from build123d import *

# Parameters (mm, degrees)
SKETCH1_R           = 7
BOSS_EXTRUDE1_DEPTH = 10


with BuildPart() as part:
    # Sketch1 → Boss-Extrude1 (new body)
    with BuildSketch(Plane.XY):
        with BuildLine():
            Line((-63.333523535, 182.443481279), (-143.333523535, 182.443481279))
            ThreePointArc((-143.333523535, 182.443481279), (-150.404591346, 179.514549091), (-153.333523535, 172.443481279))
            Line((-153.333523535, 172.443481279), (-153.333523535, -75.556518721))
            ThreePointArc((-153.333523535, -75.556518721), (-150.404591346, -82.627586533), (-143.333523535, -85.556518721))
            Line((-143.333523535, -85.556518721), (-63.333523535, -85.556518721))
            Line((-63.333523535, -85.556518721), (-63.333523535, 182.443481279))
        make_face()
        with Locations((-108.333523535, 48.443481279)):
            Circle(SKETCH1_R, mode=Mode.SUBTRACT)
        with Locations((-108.333523535, 123.443481279)):
            Circle(SKETCH1_R, mode=Mode.SUBTRACT)
        with Locations((-108.333523535, -26.556518721)):
            Circle(SKETCH1_R, mode=Mode.SUBTRACT)
    extrude(amount=BOSS_EXTRUDE1_DEPTH)


solid = part.part
Here's how the part is built. I have some questions about the finished solid (model axes, mm). Coordinates: 2 decimals unless noted, no trailing zeros. Order: outer loops, then holes, each group sorted by start corner. A loop starts at its lowest first (then second) coordinate and runs counter-clockwise, first axis right, second up.
Item 1: If we section it at B-B on z = 7.75: List the corners of the cut face in (x, y) for me.
Result sheet:
outline: (-153.33, -75.56) arc R10 ccw to (-143.33, -85.56) - (-63.33, -85.56) - (-63.33, 182.44) - (-143.33, 182.44) arc R10 ccw to (-153.33, 172.44) - close; hole circle Ø14 at (-108.33, -26.56); hole circle Ø14 at (-108.33, 48.44); hole circle Ø14 at (-108.33, 123.44)
Item 2: I need wall thicknesses on line 1 (Y direction, x = -111, z = 2.25); line 2 (Y direction, x = -113, z = 5.25); line 3 (X direction, y = -23.5, z = 5.25). Which ranges of each line are inside material? Lowest first, please.
Result sheet:
line 1: y = -85.56 to -33.03, -20.08 to 41.97, 54.92 to 116.97, 129.92 to 182.44
line 2: y = -85.56 to -31.77, -21.34 to 43.23, 53.66 to 118.23, 128.66 to 182.44
line 3: x = -153.33 to -114.63, -102.04 to -63.33
Item 3: For P1, Ø12.5, axis at x = -108.33, y = 123.44, coming from the -Z side, with a flat end and sliding along its axis, tell me the tip position at first contact or that it passes through.
Result sheet:
P1: passes through
Item 4: If we section it at A-A on y = 119.5: List the corners of the cut face in (x, z) for me, plus the area to 3 significant figures.
Result sheet:
outline: (-153.33, 0) - (-114.12, 0) - (-114.12, 10) - (-153.33, 10) - close; (-102.55, 0) - (-63.33, 0) - (-63.33, 10) - (-102.55, 10) - close
area: 784 mm2
Item 5: If we mould it in two halves opening along Y, with no side actions, what happens to faces 1 (the face through (-99, 50, 10)), 2 (the face through (-101.87, -29.24, 4.93)), 3 (the face through (-150.33, 179.59, 4.93))? For each: +Y half, -Y half, draft (parallel to the pull), parting line (faces both ways), or undercut.
Result sheet:
face 1: draft
face 2: undercut
face 3: +Y half
